CAD build for the part. Positions are in the model's coordinates, mm. Give positions to 0.01 mm unless a question says otherwise; leave off trailing zeros. Loops run counter-clockwise (first coordinate to the right, second up) from the corner with the lowest first, then second, coordinate; pieces in that order, holes last.
Item 1: Saw through at A-A on z = 12. Give the cut face in (x, y) (3 decimals), plus the area to 3 significant figures.
Item 2: Probe probe 1 along X at (y, z) = (-0.5, 13.5); probe 2 along Z at (x, y) = (-0.5, 0.35); probe 3 along X at (y, z) = (0.95, 22.5). List the from-to ranges inside material, lowest first.
Item 3: Drop a flat-ended pin along its axis: P1, Ø1, axis at x = 0.5, z = 22.5, coming from the +Y side (3 decimals). Give the stop position or say it passes through.
from build123d import *

# Parameters (mm, degrees)
BOSS_EXTRUDE1_DEPTH = 25.63
CUT_EXTRUDE1_DEPTH  = 1.25
CHAMFER1_SIZE       = 0.2
CHAMFER2_SIZE       = 0.2


with BuildPart() as part:
    # Sketch1 → Boss-Extrude1 (new body)
    with BuildSketch(Plane.XY):
        with BuildLine():
            ThreePointArc((1.807104037, 0.5), (0, 1.875), (-1.807104037, 0.5))
            Line((-1.807104037, 0.5), (1.807104037, 0.5))
        make_face()
        with BuildLine():
            Line((1.807104037, -0.5), (-1.807104037, -0.5))
            ThreePointArc((-1.807104037, -0.5), (0, -1.875), (1.807104037, -0.5))
        make_face()
        with BuildLine():
            Line((1.807104037, 0.5), (-1.807104037, 0.5))
            ThreePointArc((-1.807104037, 0.5), (-1.875, 0), (-1.807104037, -0.5))
            Line((-1.807104037, -0.5), (1.807104037, -0.5))
            ThreePointArc((1.807104037, -0.5), (1.857948475, -0.252294402), (1.875, 0))
            ThreePointArc((1.875, 0), (1.857948475, 0.252294402), (1.807104037, 0.5))
        make_face()
    extrude(amount=BOSS_EXTRUDE1_DEPTH)

    # Sketch2 → Cut-Extrude1 (cut)
    with BuildSketch(Plane.XY.offset(25.63)):
        with BuildLine():
            Line((-1.807104037, 0.5), (1.807104037, 0.5))
            ThreePointArc((1.807104037, 0.5), (1.875, 0), (1.807104037, -0.5))
            Line((1.807104037, -0.5), (-1.807104037, -0.5))
            ThreePointArc((-1.807104037, -0.5), (-1.875, 0), (-1.807104037, 0.5))
        make_face()
    extrude(amount=-CUT_EXTRUDE1_DEPTH, mode=Mode.SUBTRACT)

    # Chamfer1
    chamfer1_edges = [part.edges().sort_by_distance(p)[0] for p in [
        (0, 1.875, 25.63),
        (0, -1.875, 25.63),
    ]]
    chamfer(chamfer1_edges, length=CHAMFER1_SIZE)

    # Chamfer2
    chamfer2_edges = [part.edges().sort_by_distance(p)[0] for p in [
        (-1.807104037, 0.5, 0),
    ]]
    chamfer(chamfer2_edges, length=CHAMFER2_SIZE)


solid = part.part
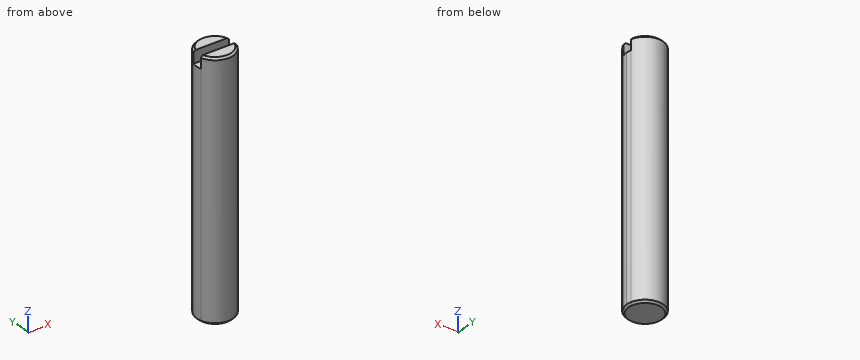
Results below:
1. outline: circle Ø3.75 at (0, 0)
1. area: 11.0 mm2
2. probe 1: x = -1.81 to 1.81
2. probe 2: z = 0 to 24.38
2. probe 3: x = -1.62 to 1.62
3. P1: stops at y = 1.875
